```python
from build123d import *

# Parameters (mm, degrees)
BOSS_EXTRUDE2_DEPTH = 10
SKETCH3_R           = 6
CUT_EXTRUDE1_DEPTH  = 10
SKETCH4_R           = 16.5
CUT_EXTRUDE2_DEPTH  = 10


with BuildPart() as part:
    # Sketch1 → Boss-Extrude2 (new body)
    with BuildSketch(Plane(origin=(0, 0, 0), x_dir=(1, 0, 0), z_dir=(0, 1, 0))):
        with BuildLine():
            Line((-171.764705882, 14.895832073), (-4.117647059, 34.756941504))
            ThreePointArc((-4.117647059, 34.756941504), (0, 35), (4.117647059, 34.756941504))
            Line((4.117647059, 34.756941504), (171.764705882, 14.895832073))
            ThreePointArc((171.764705882, 14.895832073), (184.999999986, -0.000651143), (171.763412633, -14.895985227))
            Line((171.763412633, -14.895985227), (5.118683106, -34.623678072))
            ThreePointArc((5.118683106, -34.623678072), (-0.464934327, -34.996911808), (-6.036666108, -34.475479145))
            Line((-6.036666108, -34.475479145), (-171.759908797, -14.896399599))
            ThreePointArc((-171.759908797, -14.896399599), (-184.999999806, -0.00241527), (-171.764705882, 14.895832073))
        make_face()
    extrude(amount=BOSS_EXTRUDE2_DEPTH)

    # Sketch3 → Cut-Extrude1 (cut)
    with BuildSketch(Plane(origin=(0, 10, 0), x_dir=(1, 0, 0), z_dir=(0, 1, 0))):
        with Locations((170, 0)):
            Circle(SKETCH3_R)
        with Locations((-170, 0)):
            Circle(SKETCH3_R)
        with Locations((-150, 0)):
            Circle(SKETCH3_R)
        with Locations((150, 0)):
            Circle(SKETCH3_R)
    extrude(amount=-CUT_EXTRUDE1_DEPTH, mode=Mode.SUBTRACT)

    # Sketch4 → Cut-Extrude2 (cut)
    with BuildSketch(Plane(origin=(0, 10, 0), x_dir=(1, 0, 0), z_dir=(0, 1, 0))):
        Circle(SKETCH4_R)
    extrude(amount=-CUT_EXTRUDE2_DEPTH, mode=Mode.SUBTRACT)


solid = part.part
```
Work out the finished part from the listing and answer in its coordinate system (mm). Round coordinates to 2 decimals unless told otherwise and drop trailing zeros. Write each loop counter-clockwise with the first axis right and the second up, starting at its lowest first coordinate (ties: lowest second). Pieces come first, ordered by that corner, then holes.
1) Determine the mould class of faces 1 (the face through (3, 10, 23)), 2 (the face through (3, 0, 23)), 3 (the face through (145.24, 5.07, 3.65)) for opening direction Y: pulls with the +Y half, pulls with the -Y half, needs draft (parallel to the pull), parting line crosses it, or undercut.
2) Flat-ended cylindrical pins translate along their axes: P1, Ø6, axis at x = -18, y = 8.5, coming from the +Z side; P2, Ø5, axis at x = 93, z = 7.5, coming from the -Y side; P3, Ø1, axis at x = -73.5, y = 2.5, coming from the -Z side; P4, Ø5, axis at x = -128, y = 3, coming from the -Z side. Find the tip coordinate at first contact, or state that the pin passes through.
3) Consider probe 1 along X at (y, z) = (6.75, 0); probe 2 along X at (y, z) = (8.25, 2.5); probe 3 along Z at (x, y) = (170, 7.5). Determine where each line is inside the solid, lowest interval first.
4) A cutting plane is placed at D-D on x = -150. Determine the outline of the cut face in (y, z), and give its area (3 significant figures).
5) A cutting plane is placed at C-C on z = 0. Determine the outline of the cut face in (x, y), and give its area (3 significant figures).
6) A cutting plane is placed at B-B on y = 7.5. Determine the outline of the cut face in (x, z), and give its area (3 significant figures).
7) A cutting plane is placed at A-A on x = 0. Determine the outline of the cut face in (y, z), and give its area (3 significant figures).
Entries:
1. face 1: pulls with the +Y half
1. face 2: pulls with the -Y half
1. face 3: needs draft
2. P1: stops at z = 33.42
2. P2: stops at y = 0
2. P3: stops at z = -26.6
2. P4: stops at z = -20.38
3. probe 1: x = -185 to -176, -164 to -156, -144 to -16.5, 16.5 to 144, 156 to 164, 176 to 185
3. probe 2: x = -184.79 to -175.45, -164.55 to -155.45, -144.55 to -16.31, 16.31 to 144.55, 155.45 to 164.55, 175.45 to 184.79
3. probe 3: z = -15.1 to -6, 6 to 15.1
4. outline: (0, -17.47) - (10, -17.47) - (10, -6) - (0, -6) - close; (0, 6) - (10, 6) - (10, 17.47) - (0, 17.47) - close
4. area: 229 mm2
5. outline: (-185, 0) - (-176, 0) - (-176, 10) - (-185, 10) - close; (-164, 0) - (-156, 0) - (-156, 10) - (-164, 10) - close; (-144, 0) - (-16.5, 0) - (-16.5, 10) - (-144, 10) - close; (16.5, 0) - (144, 0) - (144, 10) - (16.5, 10) - close; (156, 0) - (164, 0) - (164, 10) - (156, 10) - close; (176, 0) - (185, 0) - (185, 10) - (176, 10) - close
5. area: 2,890 mm2
6. outline: (-171.76, -14.9) - (-4.12, -34.76) arc R35 ccw to (4.12, -34.76) - (171.76, -14.9) arc R15 ccw to (171.76, 14.9) - (5.12, 34.62) arc R35 ccw to (-6.04, 34.48) - (-171.76, 14.9) arc R15 ccw to start; hole circle Ø12 at (-170, 0); hole circle Ø12 at (-150, 0); hole circle Ø33 at (0, 0); hole circle Ø12 at (150, 0); hole circle Ø12 at (170, 0)
6. area: 16,500 mm2
7. outline: (0, -35) - (10, -35) - (10, -16.5) - (0, -16.5) - close; (0, 16.5) - (10, 16.5) - (10, 35) - (0, 35) - close
7. area: 370 mm2
